Here's how the part is built. I have some questions about the finished solid (model axes, mm). Face numbers are marked on the shaded views. A direction names the side the tool comes from. Coordinates: 2 decimals unless noted, no trailing zeros. Loops run counter-clockwise (first coordinate to the right, second up) from the corner with the lowest first, then second, coordinate; pieces in that order, holes last.
```python
from build123d import *

# Parameters (mm, degrees)
CUT_EXTRUDE_1_DEPTH      = 281.922693463
CUT_EXTRUDE_1_DEPTH_BACK = 281.922693463
SKETCH_3_W               = 42.4
SKETCH_3_H               = 20
CUT_EXTRUDE_START        = 3.96072
SKETCH_4_R               = 10
CUT_EXTRUDE_2_DEPTH      = 8.000001
SKETCH_5_R               = 6.5
CUT_EXTRUDE_3_DEPTH      = 280.792780464
PATTERN_CIRCULAR_1_COUNT = 6
CHAMFER_1_SIZE           = 2


with BuildPart() as part:
    # Эскиз1 → Повернуть1 (revolve)
    with BuildSketch(Plane.XY, mode=Mode.PRIVATE) as revolve_1_sk:
        Polygon((-18.039279514, 135), (-18.039279514, 150), (-13.039279514, 150), (-13.039279514, 190), (11.960720486, 190), (11.960720486, 150), (5.960720486, 150), (5.960720486, 60), (81.960720486, 60), (81.960720486, 37.5), (-18.039279514, 37.5), (-18.039279514, 60), (-12.039279514, 60), (-12.039279514, 135), align=None)
    revolve(revolve_1_sk.sketch.rotate(Axis((-127.420307677, 0, 0), (1, 0, 0)), 90), axis=Axis((-127.420307677, 0, 0), (1, 0, 0)))

    # Эскиз3 → Вырез-Вытянуть1 (cut, two sides: drawn at the far end of the back side and taken through both)
    with BuildSketch(Plane(origin=(0, 0, 0), x_dir=(0, 0, -1), z_dir=(1, 0, 0)).offset(-CUT_EXTRUDE_1_DEPTH_BACK)):
        with Locations((-21.2, 0)):
            Rectangle(SKETCH_3_W, SKETCH_3_H)
    extrude(amount=CUT_EXTRUDE_1_DEPTH + CUT_EXTRUDE_1_DEPTH_BACK, mode=Mode.SUBTRACT)

    # Эскиз4 → Вырез-Вытянуть2 (cut)
    with BuildSketch(Plane(origin=(0, 0, 0), x_dir=(0, 0, -1), z_dir=(1, 0, 0)).offset(CUT_EXTRUDE_START)):
        with Locations(Location((0, -172.5, 0), (0, 0, 180))):
            Circle(SKETCH_4_R)
    cut_extrude_2 = extrude(amount=CUT_EXTRUDE_2_DEPTH, mode=Mode.SUBTRACT)

    # Эскиз5 → Вырез-Вытянуть3 (cut, through all)
    with BuildSketch(Plane(origin=(3.960720486, 0, 0), x_dir=(0, 0, -1), z_dir=(1, 0, 0))):
        with Locations((0, -172.5)):
            Circle(SKETCH_5_R)
    cut_extrude_3 = extrude(amount=-CUT_EXTRUDE_3_DEPTH, mode=Mode.SUBTRACT)

    # Круговой массив1: Вырез-Вытянуть2, Вырез-Вытянуть3 ×6 about axis
    pattern_circular_1_axis = Axis((0, 0, 0), (1, 0, 0))
    add([cut_extrude_2.rotate(pattern_circular_1_axis, i * 360 / PATTERN_CIRCULAR_1_COUNT) for i in range(1, PATTERN_CIRCULAR_1_COUNT)], mode=Mode.SUBTRACT)
    add([cut_extrude_3.rotate(pattern_circular_1_axis, i * 360 / PATTERN_CIRCULAR_1_COUNT) for i in range(1, PATTERN_CIRCULAR_1_COUNT)], mode=Mode.SUBTRACT)

    # Фаска1
    chamfer_1_edges = [part.edges().sort_by_distance(p)[0] for p in [
        (11.960720486, 0, -190),
        (81.960720486, 0, -60),
        (81.960720486, 0, -37.5),
        (-18.039279514, 0, -37.5),
        (-18.039279514, 0, -60),
        (-18.039279514, 0, -150),
    ]]
    chamfer(chamfer_1_edges, length=CHAMFER_1_SIZE)


solid = part.part
```
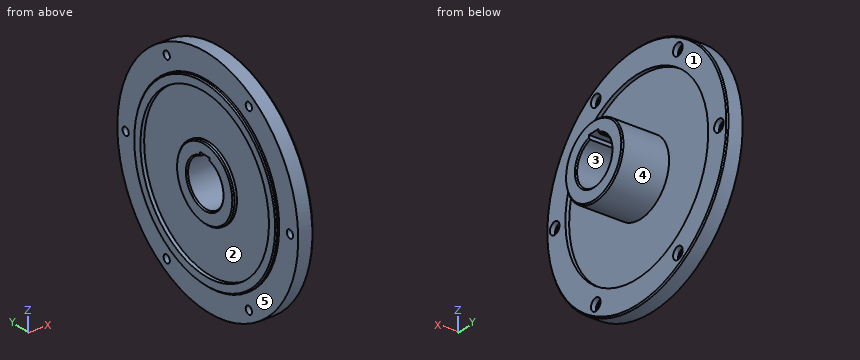
1. We'd pull the mould along Y, two halves only. Please class the marked faces 1 and 2: +Y half, -Y half, draft (parallel to the pull), parting line (faces both ways), or undercut.
2. I want a section at B-B (z = 0). Give the number of separate pieces and of enclosed holes in the cut face, then the cut area to 3 significant figures.
3. I need wall thicknesses on line 1 along Y through (x, z) = (-16, 0); line 2 along Z through (x, y) = (-5, 86); line 3 along Y through (x, z) = (-3.5, 0). Which ranges of each line are inside material? Lowest first, please.
4. I want a section at A-A (x = 44). Please give me the cut outline in (y, z).
5. For pin 1 (12 mm diameter, centred on y = 86.25, z = 149.39, fed in from +X); pin 2 (23 mm diameter, centred on y = -172.5, z = 0, fed in from -X); pin 3 (1.5 mm diameter, centred on y = 102, z = -116, fed in from +X); pin 4 (3 mm diameter, centred on x = 42.5, z = -16.5, fed in from -Y), each with a flat end and sliding along its axis, tell me the tip position at first contact or that it passes through.
6. On a 3-axis mill with a long thin cutter (end or side, diameter ignored), from which of +Z, -Z, +X, -X, +Y, -Y can I reach the whole of each face in a straight line? I mean the marked faces 3, 4 and 5. Say none if no direction works.
Response values:
1. face 1: draft
1. face 2: undercut
2. separate pieces: 4
2. enclosed holes: 0
2. area: 9,130 mm2
3. line 1: y = -150 to -135, -60 to -37.5, 37.5 to 60, 135 to 150
3. line 2: z = -169.42 to -155.88, -142.89 to 142.89, 155.88 to 169.42
3. line 3: y = -190 to -179, -166 to -37.5, 37.5 to 166, 179 to 190
4. outline: circle Ø120 at (0, 0); hole (-10, 36.14) arc R37.5 ccw (long way) to (10, 36.14) - (10, 42.4) - (-10, 42.4) - close
5. pin 1: passes through
5. pin 2: stops at x = -13.04
5. pin 3: stops at x = 11.96
5. pin 4: stops at y = -58.09
6. face 3: +X, -X
6. face 4: +X
6. face 5: -X
